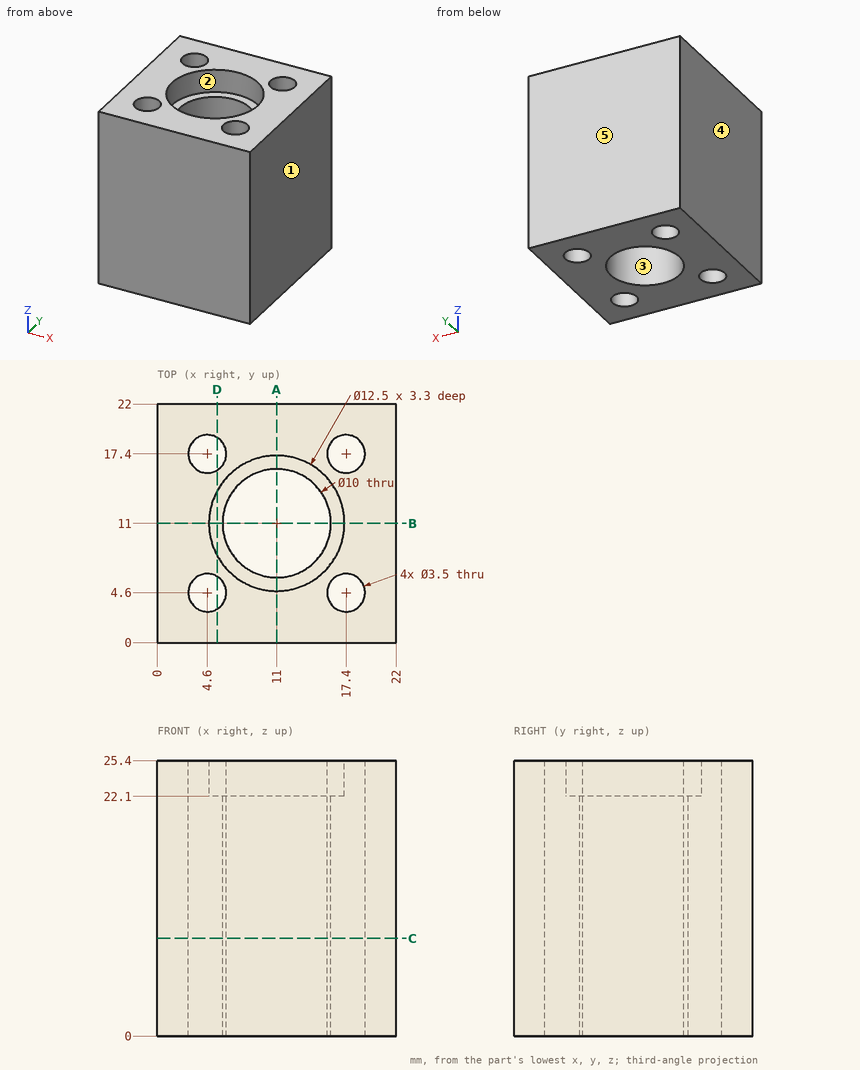
For this review, use the dimensioned drawing (mm, ordinates from the lowest corner) and the shaded views. A direction names the side the tool comes from. Coordinates: 2 decimals unless noted, no trailing zeros. Order: outer loops, then holes, each group sorted by start corner. A loop starts at its lowest first (then second) coordinate and runs counter-clockwise, first axis right, second up. Notation, with made-up numbers: (63.25, -26.75) - (109.25, -26.75) arc R20 ccw to (109.25, -8.75) - close; hole circle Ø7 at (88, -37). An arc over 180 degrees is marked (long way). Use one line per item in the form item = value.
Q1. Consider section C-C (z = 9). Give the boundary of the cut face in (x, y).
Checked values:
outline = (0, 0) - (22, 0) - (22, 22) - (0, 22) - close; hole circle Ø3.5 at (4.6, 4.6); hole circle Ø3.5 at (4.6, 17.4); hole circle Ø10 at (11, 11); hole circle Ø3.5 at (17.4, 4.6); hole circle Ø3.5 at (17.4, 17.4)
Q2. Consider section D-D (x = 5.5). Give the boundary of the cut face in (y, z), then the cut area to 3 significant figures.
Checked values:
outline = (0, 0) - (3.1, 0) - (3.1, 25.4) - (0, 25.4) - close; (6.1, 0) - (15.9, 0) - (15.9, 25.4) - (13.97, 25.4) - (13.97, 22.1) - (8.03, 22.1) - (8.03, 25.4) - (6.1, 25.4) - close; (18.9, 0) - (22, 0) - (22, 25.4) - (18.9, 25.4) - close
area = 387 mm2
Q3. Draft analysis for pull direction Y (two halves, no side actions). For the marked faces 3, 4 and 5, state which applies: +Y half, -Y half, draft (parallel to the pull), parting line (faces both ways), or undercut.
Checked values:
face_3 = undercut
face_4 = draft
face_5 = +Y half
Q4. For probe 1 along X at (y, z) = (4.6, 18); probe 2 along Y at (x, z) = (11, 24.25), list the stretches that pass through material, from the lowest coordinate up. Write a range as from..to.
Checked values:
probe_1 = 0..2.85, 6.35..15.65, 19.15..22
probe_2 = 0..4.75, 17.25..22
Q5. Consider section A-A (x = 11). Give the boundary of the cut face in (y, z), then the cut area to 3 significant figures.
Checked values:
outline = (0, 0) - (6, 0) - (6, 22.1) - (4.75, 22.1) - (4.75, 25.4) - (0, 25.4) - close; (16, 0) - (22, 0) - (22, 25.4) - (17.25, 25.4) - (17.25, 22.1) - (16, 22.1) - close
area = 297 mm2
Q6. For P1, Ø11, axis at x = 11, y = 11, coming from the +Z side, flat-tipped, find the tip position at first contact; note if it passes through.
Checked values:
P1 = 22.1
Q7. For the marked faces 1 and 2, list the 3-axis set-ups (+Z, -Z, +X, -X, +Y, -Y) from which the entire face can be reached by the end or side of a thin tool; tool diameter is ignored.
Checked values:
face_1 = +Z, -Z, +X, +Y, -Y
face_2 = +Z
